Check sheet for the drawn part. Datum: minimum x, y, z corner. Units: mm. A direction names the side the tool comes from. Round coordinates to 2 decimals unless told otherwise and drop trailing zeros. Write each loop counter-clockwise with the first axis right and the second up, starting at its lowest first coordinate (ties: lowest second). Pieces come first, ordered by that corner, then holes. Notation, with made-up numbers: (62.5, 85) -> (120.5, 85) arc R13 cw to (120.5, 105) -> close; hole circle Ø9 at (63, -37.75). An arc over 180 degrees is marked (long way). One line per item, written item: value. Start each with the question number.
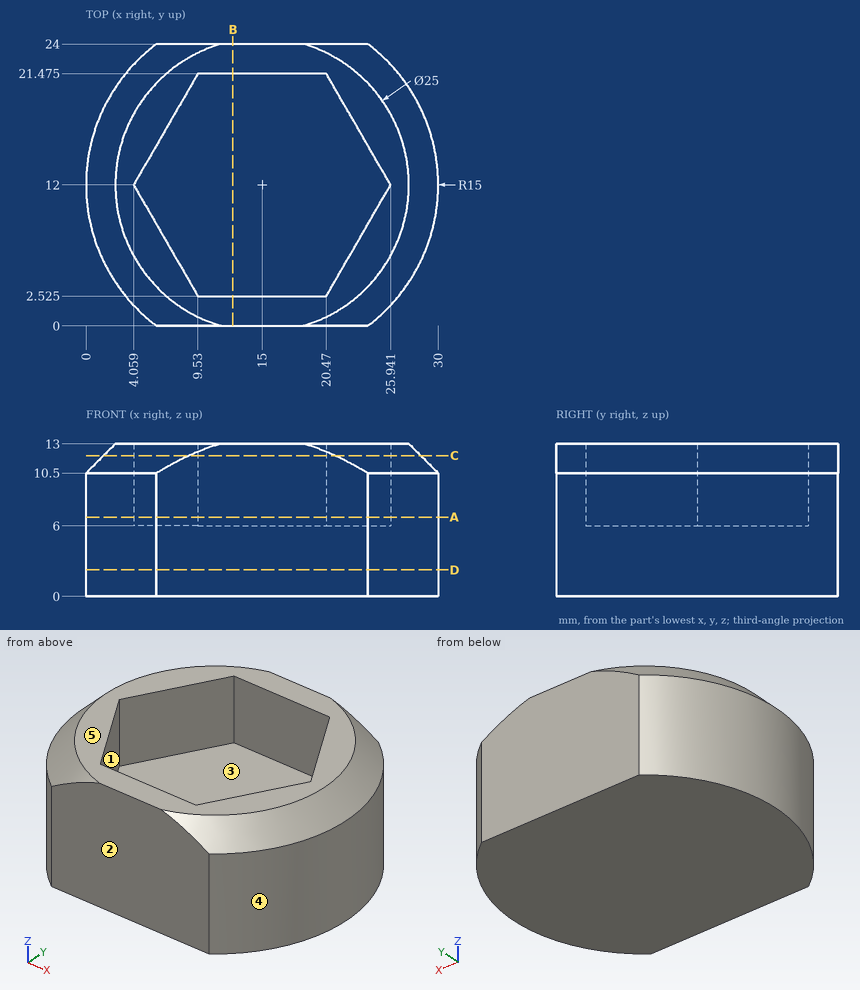
1. Cross-section at C-C (z = 12). Record the cut outline in (x, y) (1 decimal).
2. Access from +Z, -Z, +X, -X, +Y, -Y to the whole of each face (thin tool, end or side, straight path). Record for the marked faces 1 and 2.
3. Cross-section at B-B (x = 12.5). Record the cut outline in (y, z) (1 decimal).
4. Material ranges on probe 1 along Y at (x, z) = (19, 8.75) (1 decimal); probe 2 along Z at (x, y) = (17.5, 9.5); probe 3 along X at (y, z) = (3.5, 9.5) (1 decimal), recorded low to high.
5. Release check for a two-part mould opening along X. For the marked faces 3, 4 and 5 record: +X half, -X half, draft (parallel to the pull), parting line (faces both ways), or undercut.
6. Cross-section at A-A (z = 6.75). Record the cut outline in (x, y) (1 decimal), plus the area to 3 significant figures.
7. Cross-section at D-D (z = 2.25). Record the cut outline in (x, y).
Working result:
1. outline: (8.8, 0) -> (21.2, 0) arc R13.5 ccw to (21.2, 24) -> (8.8, 24) arc R13.5 ccw to start; hole (4.1, 12) -> (9.5, 2.5) -> (20.5, 2.5) -> (25.9, 12) -> (20.5, 21.5) -> (9.5, 21.5) -> close
2. face 1: +Z
2. face 2: +Z, -Z, +X, -X, -Y
3. outline: (0, 0) -> (24, 0) -> (24, 13) -> (21.5, 13) -> (21.5, 6) -> (2.5, 6) -> (2.5, 13) -> (0, 13) -> close
4. probe 1: y = 0 to 2.5, 21.5 to 24
4. probe 2: z = 0 to 6
4. probe 3: x = 2.6 to 9, 21 to 27.4
5. face 3: undercut
5. face 4: +X half
5. face 5: draft
6. outline: (6, 0) -> (24, 0) arc R15 ccw to (24, 24) -> (6, 24) arc R15 ccw to start; hole (4.1, 12) -> (9.5, 2.5) -> (20.5, 2.5) -> (25.9, 12) -> (20.5, 21.5) -> (9.5, 21.5) -> close
6. area: 322 mm^2
7. outline: (6, 0) -> (24, 0) arc R15 ccw to (24, 24) -> (6, 24) arc R15 ccw to start
